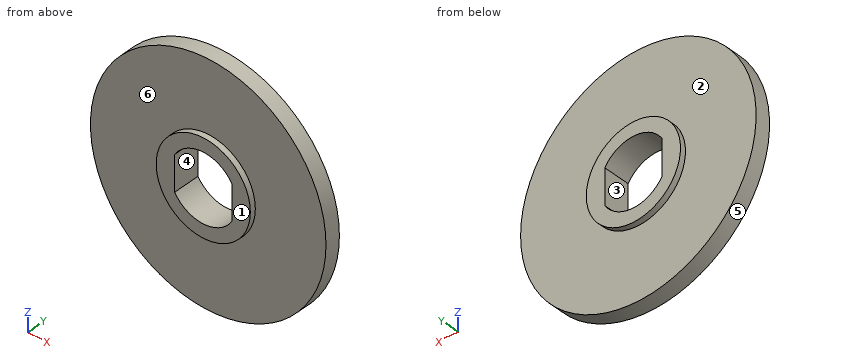
from build123d import *

# Parameters (mm, degrees)
SKETCH1_R           = 7
BOSS_EXTRUDE1_DEPTH = 2
SKETCH1_3_R         = 17.5
SKETCH1_3_R_2       = 7
BOSS_EXTRUDE2_DEPTH = 1.15


with BuildPart() as part:
    # Sketch1 → Boss-Extrude1 (new, symmetric)
    with BuildSketch(Plane(origin=(0, 0, 0), x_dir=(1, 0, 0), z_dir=(0, 1, 0))):
        Circle(SKETCH1_R)
        with BuildLine():
            Line((-4.25, -2.633913438), (-4.25, 2.633913438))
            ThreePointArc((-4.25, 2.633913438), (0, 5), (4.25, 2.633913438))
            Line((4.25, 2.633913438), (4.25, -2.633913438))
            ThreePointArc((4.25, -2.633913438), (0, -5), (-4.25, -2.633913438))
        make_face(mode=Mode.SUBTRACT)
    extrude(amount=BOSS_EXTRUDE1_DEPTH, both=True)

    # Sketch1<3> → Boss-Extrude2 (add, symmetric)
    with BuildSketch(Plane(origin=(0, 0, 0), x_dir=(1, 0, 0), z_dir=(0, 1, 0))):
        Circle(SKETCH1_3_R)
        Circle(SKETCH1_3_R_2, mode=Mode.SUBTRACT)
    extrude(amount=BOSS_EXTRUDE2_DEPTH, both=True)


solid = part.part
Geometry: final body of the model. Coordinates: model frame, mm. Face numbers are marked on the shaded views. A direction names the side the tool comes from. Give positions to 0.01 mm unless a question says otherwise; leave off trailing zeros. Write each loop counter-clockwise with the first axis right and the second up, starting at its lowest first coordinate (ties: lowest second). Pieces come first, ordered by that corner, then holes.
(1) Access query for the marked faces 1, 2 and 3. Directions: +Z, -Z, +X, -X, +Y, -Y. A direction counts if a zero-diameter tool reaches every point of the face in a straight line with its end or side. Return the directions, or none.
(2) Cut plane C-C, the plane y = 0.2. Return loops of the section in (x, z), then the cut area to 3 significant figures.
(3) Mould query, pull axis Z, two halves, no side actions, for the marked faces 4, 5 and 6. Classes: released by +Z, released by -Z, zero draft, split by the parting line, or undercut.
(4) First-contact query: P1, Ø1, axis at y = 1, z = -7, coming from the +X side; P2, Ø1.5, axis at x = 8.5, z = -8.5, coming from the -Y side; P3, Ø1.5, axis at y = -1, z = -5, coming from the +X side. Flat tips, straight axial feed; report the tip coordinate or a pass-through.
(5) Ray query, line 1 (Y direction, x = -6, z = -4.5); line 2 (Z direction, x = -2, y = 1.8); line 3 (Z direction, x = -3, y = 0.85). Return the intervals inside material, ascending.
(6) Cut plane D-D, the plane z = 14.5. Return loops of the section in (x, y), then the cut area to 3 significant figures.
(7) Cut plane A-A, the plane z = 0. Return loops of the section in (x, y).
(8) Cut plane B-B, the plane x = 0. Return loops of the section in (y, z).
Values follow:
1. face 1: +Z, -Z, +X, -X, -Y
1. face 2: +Y
1. face 3: +Y, -Y
2. outline: circle Ø35 at (0, 0); hole (-4.25, -2.63) arc R5 ccw to (4.25, -2.63) - (4.25, 2.63) arc R5 ccw to (-4.25, 2.63) - close
2. area: 889 mm2
3. face 4: undercut
3. face 5: split by the parting line
3. face 6: zero draft
4. P1: stops at x = 16.25
4. P2: stops at y = -1.15
4. P3: stops at x = 16.98
5. line 1: y = -1.15 to 1.15
5. line 2: z = -6.71 to -4.58, 4.58 to 6.71
5. line 3: z = -17.24 to -4, 4 to 17.24
6. outline: (-9.8, -1.15) - (9.8, -1.15) - (9.8, 1.15) - (-9.8, 1.15) - close
6. area: 45.1 mm2
7. outline: (-17.5, -1.15) - (-7, -1.15) - (-7, -2) - (-4.25, -2) - (-4.25, 2) - (-7, 2) - (-7, 1.15) - (-17.5, 1.15) - close; (4.25, -2) - (7, -2) - (7, -1.15) - (17.5, -1.15) - (17.5, 1.15) - (7, 1.15) - (7, 2) - (4.25, 2) - close
8. outline: (-2, -7) - (-1.15, -7) - (-1.15, -17.5) - (1.15, -17.5) - (1.15, -7) - (2, -7) - (2, -5) - (-2, -5) - close; (-2, 5) - (2, 5) - (2, 7) - (1.15, 7) - (1.15, 17.5) - (-1.15, 17.5) - (-1.15, 7) - (-2, 7) - close
